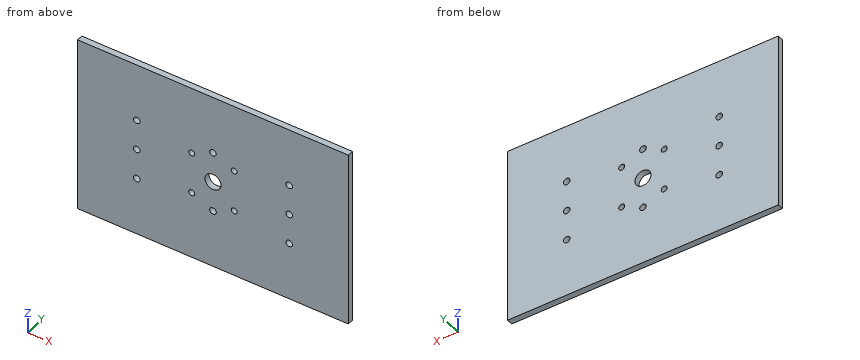
```python
from build123d import *

# Parameters (mm, degrees)
F0_W     = 135
F0_H     = 90
F1_DEPTH = 3
F2_R     = 1.65
F2_R_2   = 1.5
F2_R_3   = 4
F3_DEPTH = 3.001


with BuildPart() as f1:
    # F0 (on Front) → F1 (new body)
    with BuildSketch(Plane.XZ):
        Rectangle(F0_W, F0_H)
    extrude(amount=F1_DEPTH)

    # F2 (on face) → F3 (cut, through all)
    with BuildSketch(Plane.XZ.offset(3)):
        with Locations((0, 15.5)):
            Circle(F2_R)
        with Locations((0, -15.5)):
            Circle(F2_R)
        with Locations((38, 0)):
            Circle(F2_R)
        with Locations((-38, 0)):
            Circle(F2_R)
        with Locations((-38, 15.5)):
            Circle(F2_R)
        with Locations((-38, -15.5)):
            Circle(F2_R)
        with Locations((38, 15.5)):
            Circle(F2_R)
        with Locations((38, -15.5)):
            Circle(F2_R)
        with Locations((10.606602, 10.606602)):
            Circle(F2_R_2)
        with Locations((-10.606602, -10.606602)):
            Circle(F2_R_2)
        with Locations((-10.606602, 10.606602)):
            Circle(F2_R_2)
        with Locations((10.606602, -10.606602)):
            Circle(F2_R_2)
        Circle(F2_R_3)
    extrude(amount=-F3_DEPTH, mode=Mode.SUBTRACT)


solid = f1.part
```
Input: part model. Units: mm. Frame: model coordinates. Give positions to 0.01 mm unless a question says otherwise; leave off trailing zeros. Write each loop counter-clockwise with the first axis right and the second up, starting at its lowest first coordinate (ties: lowest second). Pieces come first, ordered by that corner, then holes. Notation, with made-up numbers: (3.25, 55.5) - (26.25, 55.5) arc R14 cw to (26.25, 70.5) - close; hole circle Ø8 at (55, -8.75). An arc over 180 degrees is marked (long way). Write item = value, one per line. Start each with the question number.
1. Section query A-A, the plane x = 0. Output: boundary loops of the cut face in (y, z), then the cut area to 3 significant figures.
2. Section query B-B, the plane z = -15.5. Output: boundary loops of the cut face in (x, y).
3. Ray query, L1, parallel to Z at x = 0, y = -2.4; L2, parallel to Z at x = -38, y = -1.15; L3, parallel to Z at x = -11, y = -1.95. Return the intervals inside material, ascending.
Check sheet entries:
q1.outline = (-3, -45) - (0, -45) - (0, -17.15) - (-3, -17.15) - close; (-3, -13.85) - (0, -13.85) - (0, -4) - (-3, -4) - close; (-3, 4) - (0, 4) - (0, 13.85) - (-3, 13.85) - close; (-3, 17.15) - (0, 17.15) - (0, 45) - (-3, 45) - close
q1.area = 226 mm2
q2.outline = (-67.5, -3) - (-39.65, -3) - (-39.65, 0) - (-67.5, 0) - close; (-36.35, -3) - (-1.65, -3) - (-1.65, 0) - (-36.35, 0) - close; (1.65, -3) - (36.35, -3) - (36.35, 0) - (1.65, 0) - close; (39.65, -3) - (67.5, -3) - (67.5, 0) - (39.65, 0) - close
q3.L1 = -45 to -17.15, -13.85 to -4, 4 to 13.85, 17.15 to 45
q3.L2 = -45 to -17.15, -13.85 to -1.65, 1.65 to 13.85, 17.15 to 45
q3.L3 = -45 to -12.05, -9.16 to 9.16, 12.05 to 45
